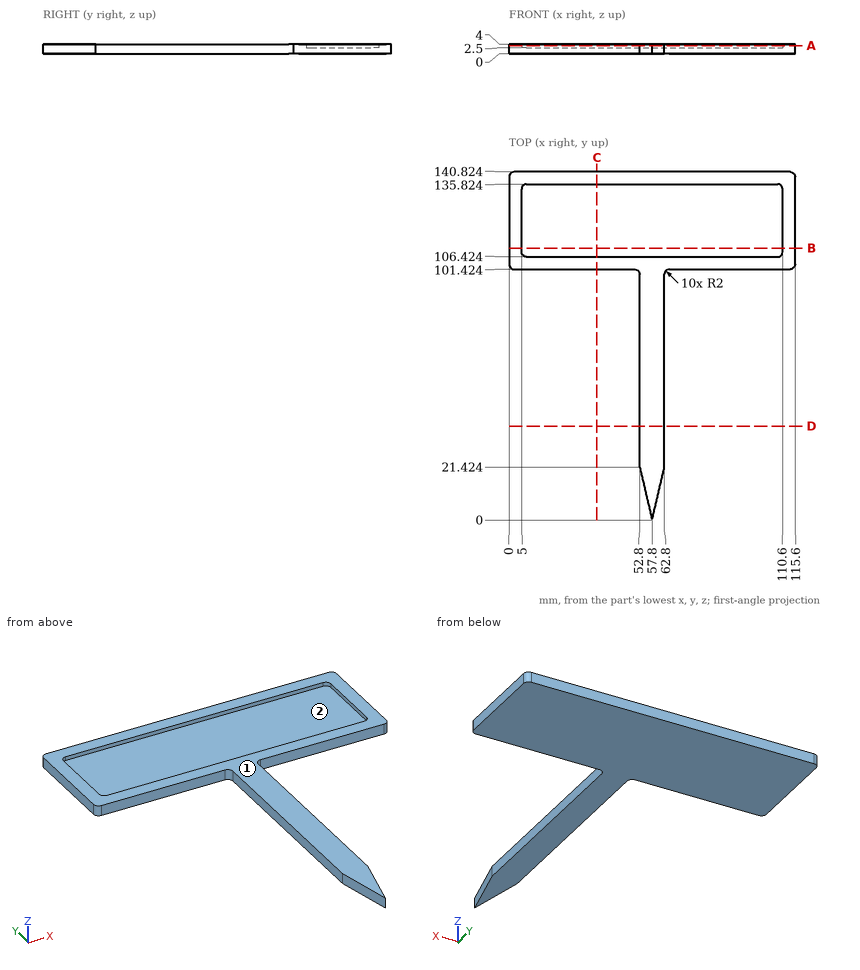
Geometry check sheet. Reference: drawing and pictorial views, mm from the part's lowest x, y, z. Give positions to 0.01 mm unless a question says otherwise; leave off trailing zeros. Order: outer loops, then holes, each group sorted by start corner. A loop starts at its lowest first (then second) coordinate and runs counter-clockwise, first axis right, second up. Notation, with made-up numbers: M 38,33.5 L 78,33.5 A15 ccw 78,49.5 Z; hole C 58,82.25 d7. An arc over 180 degrees is marked long. Return JSON: item names as keys, results as strings. Group by question number.
1) Section check D-D on y = 38. Record the cut outline in (x, z).
2) Section check C-C on x = 35.5. Record the cut outline in (y, z).
3) Scan lines: line 1 (Y direction, x = 72, z = 3.6); line 2 (X direction, y = 90.5, z = 0.8); line 3 (Z direction, x = 10, y = 133). Record each from-to range of solid material in increasing order.
4) Section check A-A on z = 3.3. Record the cut outline in (x, y), and give its area (3 significant figures).
5) Section check B-B on y = 110. Record the cut outline in (x, z).
6) Go/stop test with flat-tipped pins: pin 1 Ø2 at (x, y) = (63, 57.5) entering from -Z; pin 2 Ø1 at (x, z) = (15, 1) entering from -Y; pin 3 Ø23.5 at (x, y) = (36, 123.5) entering from +Z; pin 4 Ø2 at (y, z) = (75, 2) entering from -X. Record where each tip stops, or that it passes through.
7) Mould release check, pull along Y, two halves, no side actions. Record for the marked faces 1 and 2: pulls with the +Y half, pulls with the -Y half, needs draft (parallel to the pull), parting line crosses it, or undercut.
Answer block:
{
 "1": {"outline": "M 52.8,0 L 62.8,0 L 62.8,4 L 52.8,4 Z"},
 "2": {"outline": "M 101.42,0 L 140.82,0 L 140.82,4 L 135.82,4 L 135.82,2.5 L 106.42,2.5 L 106.42,4 L 101.42,4 Z"},
 "3": {"line 1": "y = 101.42 to 106.42, 135.82 to 140.82", "line 2": "x = 52.8 to 62.8", "line 3": "z = 0 to 2.5"},
 "4": {"outline": "M 0,103.42 A2 ccw 2,101.42 L 50.8,101.42 A2 cw 52.8,99.42 L 52.8,21.42 L 57.8,0 L 62.8,21.42 L 62.8,99.42 A2 cw 64.8,101.42 L 113.6,101.42 A2 ccw 115.6,103.42 L 115.6,138.82 A2 ccw 113.6,140.82 L 2,140.82 A2 ccw 0,138.82 Z; hole M 5,108.42 A2 ccw 7,106.42 L 108.6,106.42 A2 ccw 110.6,108.42 L 110.6,133.82 A2 ccw 108.6,135.82 L 7,135.82 A2 ccw 5,133.82 Z", "area": "2,360 mm^2"},
 "5": {"outline": "M 0,0 L 115.6,0 L 115.6,4 L 110.6,4 L 110.6,2.5 L 5,2.5 L 5,4 L 0,4 Z"},
 "6": {"pin 1": "stops at z = 0", "pin 2": "stops at y = 101.42", "pin 3": "stops at z = 2.5", "pin 4": "stops at x = 52.8"},
 "7": {"face 1": "needs draft", "face 2": "undercut"}
}
